Autodesk Inventor part; units mm, degrees
ref_plane "РабПлоскость4" through (-23, -29.9, -1) normal (0, -1, 0) x (1, 0, 0)
ref_plane "РабПлоскость8" through (0, 0, -1) normal (0, 0, -1) x (-1, 0, 0)
ref_plane "YZ Plane" through (0, 0, 0) normal (1, 0, 0) x (0, 1, 0)
sketch "Эскиз1" plane through (0, 0, 0) normal (0, 0, 1) x (1, 0, 0)
  line L0 (16.9838, 20.6364) -> (20.6364, 16.9838)
  arc A0 (16.9838, 20.6364) -> (16.3474, 20.9) centre (16.3474, 20) ccw
  line L1 (-16.3474, 20.9) -> (16.3474, 20.9)
  arc A1 (-16.3474, 20.9) -> (-16.9838, 20.6364) centre (-16.3474, 20) ccw
  line L2 (-20.6364, 16.9838) -> (-16.9838, 20.6364)
  arc A2 (-20.6364, 16.9838) -> (-20.9, 16.3474) centre (-20, 16.3474) ccw
  line L3 (-20.9, -16.3474) -> (-20.9, 16.3474)
  arc A3 (-20.9, -16.3474) -> (-20.6364, -16.9838) centre (-20, -16.3474) ccw
  line L4 (-16.9838, -20.6364) -> (-20.6364, -16.9838)
  arc A4 (-16.9838, -20.6364) -> (-16.3474, -20.9) centre (-16.3474, -20) ccw
  line L5 (16.3474, -20.9) -> (-16.3474, -20.9)
  arc A5 (16.3474, -20.9) -> (16.9838, -20.6364) centre (16.3474, -20) ccw
  line L6 (20.6364, -16.9838) -> (16.9838, -20.6364)
  arc A6 (20.6364, -16.9838) -> (20.9, -16.3474) centre (20, -16.3474) ccw
  line L7 (20.9, 16.3474) -> (20.9, -16.3474)
  arc A7 (20.9, 16.3474) -> (20.6364, 16.9838) centre (20, 16.3474) ccw
  circle A8 centre (15.5574, -15.5574) radius 1.45
  circle A9 centre (0, 0) radius 11
  circle A10 centre (-15.5574, -15.5574) radius 1.45
  circle A11 centre (-15.5574, 15.5574) radius 1.45
  circle A12 centre (15.5574, 15.5574) radius 1.45
  point P0 (0, 0)
extrude "Выдавливание1" add sketch "Эскиз1" along normal blind 3
sketch "Эскиз2" plane through (0, 0, 3) normal (0, 0, 1) x (1, 0, 0)
  line L0 (16.3474, 20.9) -> (-16.3474, 20.9) construction
  line L1 (-30, -20.9) -> (30, -20.9)
  line L2 (30, -20.9) -> (30, 20.9)
  line L3 (30, 20.9) -> (-30, 20.9)
  line L4 (-30, 20.9) -> (-30, -20.9)
  circle A0 centre (0, 0) radius 11 construction
  line L5 (-30, -20.9) -> (30, 20.9) construction
  line L6 (30, -20.9) -> (-30, 20.9) construction
  line L7 (-30, -20.9) -> (30, -20.9)
  line L8 (30, -20.9) -> (30, -48.9)
  line L9 (30, -48.9) -> (-30, -48.9)
  line L10 (-30, -48.9) -> (-30, -20.9)
  line L11 (-16.9838, 20.6364) -> (-20.6364, 16.9838)
  arc A1 (-20.6364, 16.9838) -> (-20.9, 16.3474) centre (-20, 16.3474) ccw
  line L12 (-20.9, 16.3474) -> (-20.9, -16.3474)
  arc A2 (-20.9, -16.3474) -> (-20.6364, -16.9838) centre (-20, -16.3474) ccw
  line L13 (-20.6364, -16.9838) -> (-16.9838, -20.6364)
  arc A3 (-16.9838, -20.6364) -> (-16.3474, -20.9) centre (-16.3474, -20) ccw
  line L14 (-16.3474, -20.9) -> (16.3474, -20.9)
  arc A4 (16.3474, -20.9) -> (16.9838, -20.6364) centre (16.3474, -20) ccw
  line L15 (16.9838, -20.6364) -> (20.6364, -16.9838)
  arc A5 (20.6364, -16.9838) -> (20.9, -16.3474) centre (20, -16.3474) ccw
  line L16 (20.9, -16.3474) -> (20.9, 16.3474)
  arc A6 (20.9, 16.3474) -> (20.6364, 16.9838) centre (20, 16.3474) ccw
  line L17 (20.6364, 16.9838) -> (16.9838, 20.6364)
  arc A7 (16.9838, 20.6364) -> (16.3474, 20.9) centre (16.3474, 20) ccw
  line L18 (16.3474, 20.9) -> (-16.3474, 20.9)
  arc A8 (-16.3474, 20.9) -> (-16.9838, 20.6364) centre (-16.3474, 20) ccw
  circle A9 centre (0, 0) radius 11 construction
  circle A10 centre (15.5574, 15.5574) radius 1.45 construction
  circle A11 centre (-15.5574, 15.5574) radius 1.45 construction
  circle A12 centre (-15.5574, -15.5574) radius 1.45 construction
  circle A13 centre (15.5574, -15.5574) radius 1.45 construction
  dimension "d4" = 60
  dimension "d5" = 60
  dimension "d6" = 28
extrude "Выдавливание2" add sketch "Эскиз2" against normal blind 8
ref_plane "РабПлоскость4" through (-23, -29.9, -1) normal (0, -1, 0) x (1, 0, 0)
chamfer "Фаска1" distance 4 angle 45 2 edges at (30, -48.9, -1) (-30, -48.9, -1)
chamfer "Фаска2" distance 8 angle 45 2 edges at (30, 20.9, -1) (-30, 20.9, -1)
sketch "Эскиз14" plane through (-30, -44.9, -5) normal (-1, 0, 0) x (0, 0, 1)
  line L0 (0, 57.8) -> (8, 57.8) construction
  line L1 (0, 0) -> (0, 57.8) construction
  line L2 (8, 0) -> (0, 0) construction
  line L3 (8, 57.8) -> (8, 0) construction
  line L4 (8, 57.8) -> (0, 57.8)
  line L5 (4, 57.8) -> (4, 0) construction
  line L6 (8, 0) -> (0, 0)
  circle A0 centre (4, 47.8) radius 2
  circle A1 centre (4, 33.8) radius 2
  dimension "d107" = 4
  dimension "d108" = 4
  dimension "d109" = 10
  dimension "d113" = 14
extrude "Выдавливание13" cut sketch "Эскиз14" against normal blind 6
sketch "Эскиз25" plane through (0, 0, 3) normal (0, 0, 1) x (1, 0, 0)
  line L0 (-20, -42.7) -> (20, -42.7)
  line L1 (20, -42.7) -> (20, -45.9)
  line L2 (20, -45.9) -> (-20, -45.9)
  line L3 (-20, -45.9) -> (-20, -42.7)
  line L4 (-20, -42.7) -> (20, -45.9) construction
  line L5 (20, -42.7) -> (-20, -45.9) construction
  line L6 (-26, -48.9) -> (26, -48.9) construction
  line L7 (26, -48.9) -> (-26, -48.9)
  line L8 (0, -48.9) -> (0, 20.9) construction
  line L9 (16.3474, 20.9) -> (-16.3474, 20.9) construction
  point P0 (0, 0)
  point P1 (0, -44.3)
  dimension "d170" = 40
  dimension "d171" = 3.2
  dimension "d172" = 3
extrude "Выдавливание25" cut sketch "Эскиз25" against normal blind 8
sketch "Эскиз27" plane through (-26, -48.9, 3) normal (0, -1, 0) x (1, 0, 0)
  line L0 (0, -8) -> (0, 0) construction
  line L1 (52, 0) -> (52, -8) construction
  line L2 (0, -4) -> (52, -4) construction
  circle A0 centre (16, -4) radius 1.1
  line L3 (46, 0) -> (46, -8) construction
  line L4 (6, 0) -> (46, 0) construction
  line L5 (46, 0) -> (46, -8) construction
  line L6 (46, -8) -> (6, -8) construction
  line L7 (6, -8) -> (6, 0) construction
  line L8 (6, 0) -> (46, -8) construction
  line L9 (46, 0) -> (6, -8) construction
  circle A1 centre (36, -4) radius 1.1
  point P0 (26, -4)
  dimension "d177" = 2.2
  dimension "d178" = 10
  dimension "d179" = 2.2
  dimension "d180" = 10
extrude "Выдавливание26" cut sketch "Эскиз27" against normal blind 14
sketch "Эскиз28" plane through (0, 0, 3) normal (0, 0, 1) x (1, 0, 0)
  line L0 (20, -45.9) -> (-20, -45.9) construction
  line L1 (-20, -45.9) -> (-20, -42.7) construction
  line L2 (-20, -42.7) -> (20, -42.7) construction
  line L3 (20, -42.7) -> (20, -45.9) construction
  line L4 (-26, -48.9) -> (26, -48.9)
  line L5 (-13, -48.9) -> (-7, -48.9)
  line L6 (-7, -48.9) -> (-7, -38.9)
  line L7 (-7, -38.9) -> (-13, -38.9)
  line L8 (-13, -38.9) -> (-13, -48.9)
  line L9 (-10, -38.9) -> (-10, -48.9) construction
  point P0 (0, 0)
  point P1 (-10, -43.9)
  point P2 (-20, -44.3)
  dimension "d183" = 6
  dimension "d184" = 10
  dimension "d185" = 10
extrude "Выдавливание27" cut sketch "Эскиз28" against normal blind 1.5
ref_plane "РабПлоскость8" through (0, 0, -1) normal (0, 0, -1) x (-1, 0, 0)
mirror "Зеркальное отражение4" about plane through (0, 0, 0) normal (1, 0, 0) of "Выдавливание27"
mirror "Зеркальное отражение5" about plane through (0, 0, -1) normal (0, 0, -1) of "Выдавливание27", "Зеркальное отражение4"
sketch "Эскиз29" plane through (0, 0, 1.5) normal (0, 0, 1) x (1, 0, 0)
  line L0 (-13, -38.9) -> (-7, -38.9) construction
  line L1 (-13, -42.7) -> (-13, -38.9) construction
  line L2 (7, -42.7) -> (7, -38.9) construction
  line L3 (7, -38.9) -> (13, -38.9) construction
  line L4 (-13, -38.9) -> (-7, -38.9)
  line L5 (-10, -38.9) -> (-10, -42.7) construction
  line L6 (-12, -39.9) -> (-8, -39.9)
  line L7 (-8, -39.9) -> (-8, -41.5)
  line L8 (-8, -41.5) -> (-12, -41.5)
  line L9 (-12, -41.5) -> (-12, -39.9)
  line L10 (-12, -39.9) -> (-8, -41.5) construction
  line L11 (-8, -39.9) -> (-12, -41.5) construction
  line L12 (-13, -42.7) -> (-7, -42.7)
  line L13 (7, -48.9) -> (-7, -48.9) construction
  line L14 (0, -48.9) -> (0, -38.1038) construction
  line L15 (12, -39.9) -> (8, -39.9)
  line L16 (8, -39.9) -> (8, -41.5)
  line L17 (8, -41.5) -> (12, -41.5)
  line L18 (12, -41.5) -> (12, -39.9)
  point P0 (0, 0)
  point P1 (-10, -40.7)
  dimension "d188" = 4
  dimension "d189" = 1.6
  dimension "d190" = 1.2
extrude "Выдавливание28" cut sketch "Эскиз29" against normal blind 10
properties part number "каретка_м2_без_м"
Check sheet for the modelled part. Datum: model origin and axes. Units: mm. A direction names the side the tool comes from. Give positions to 0.01 mm unless a question says otherwise; leave off trailing zeros. Loops run counter-clockwise (first coordinate to the right, second up) from the corner with the lowest first, then second, coordinate; pieces in that order, holes last. Notation, with made-up numbers: M 34,-5.75 L 40,-5.75 A28 cw 40,17.25 Z; hole C 47.5,87 d8. An arc over 180 degrees is marked long. Return JSON: item names as keys, results as strings. Group by question number.
1. Cross-section at A-A on x = -14. Record the boundary of the cut face in (y, z).
2. Tool access check on faces 4 (the flat face through (-7, -47, -4)), 5 (the flat face through (-8.7, -39.9, -1)), 6 (the flat face through (-10, -42, 1.5)). Record the directions out of +Z, -Z, +X, -X, +Y, -Y that give a thin tool (end or side, any length) a straight path to the whole face; none if there is none.
3. Mould release check, pull along Z, two halves, no side actions. Record for faces 1 (the flat face through (-10, -47, -3.5)), 2 (the flat face through (13, -47, -4)), 3 (the cylindrical face through (-8.95, -37.44, -0.67)): released by +Z, released by -Z, zero draft, split by the parting line, or undercut.
4. Cross-section at D-D on y = -12. Record the boundary of the cut face in (x, z), plus the area to 3 significant figures.
5. Thickness scan on L1, parallel to Z at x = 10, y = -37.4; L2, parallel to Z at x = 10, y = -48; L3, parallel to Y at x = 16, z = 0.5. Record the ranges inside material, lowest first.
6. Go/stop test with flat-tipped pins: pin 1 (1.6 mm diameter, centred on y = -47.5, z = -4, fed in from -X); pin 2 (1.1 mm diameter, centred on x = -9, y = -40, fed in from +Z); pin 3 (1.6 mm diameter, centred on y = -46.5, z = 2.5, fed in from -X). Record where each tip stops, or that it passes through.
7. Cross-section at C-C on x = 10. Record the boundary of the cut face in (y, z), plus the area to 3 significant figures.
8. Cross-section at B-B on y = 2.9. Record the boundary of the cut face in (x, z).
Return value:
{
 "1": {"outline": "M -48.9,-5 L -45.9,-5 L -45.9,3 L -48.9,3 Z; M -42.7,-5 L 20.9,-5 L 20.9,3 L -42.7,3 Z"},
 "2": {"face 4": "-Z, -Y", "face 5": "+Z, -Z", "face 6": "+Z, -Y"},
 "3": {"face 1": "released by -Z", "face 2": "zero draft", "face 3": "undercut"},
 "4": {"outline": "M -30,-5 L 30,-5 L 30,3 L -30,3 L -30,0.79 L -24,0.79 L -24,-2.79 L -30,-2.79 Z", "area": "459 mm^2"},
 "5": {"L1": "-5 to -2.1, 0.1 to 3", "L2": "-3.5 to -2.1, 0.1 to 1.5", "L3": "-48.9 to -45.9, -42.7 to 20.9"},
 "6": {"pin 1": "x = -28.2", "pin 2": "z = 1.5", "pin 3": "x = -29.2"},
 "7": {"outline": "M -48.9,-3.5 L -45.9,-3.5 L -45.9,-2.1 L -48.9,-2.1 Z; M -48.9,0.1 L -45.9,0.1 L -45.9,1.5 L -48.9,1.5 Z; M -42.7,-3.5 L -41.5,-3.5 L -41.5,-2.1 L -42.7,-2.1 Z; M -42.7,0.1 L -41.5,0.1 L -41.5,1.5 L -42.7,1.5 Z; M -39.9,-3.5 L -38.9,-3.5 L -38.9,-5 L 20.9,-5 L 20.9,3 L -38.9,3 L -38.9,1.5 L -39.9,1.5 L -39.9,0.1 L -34.9,0.1 L -34.9,-2.1 L -39.9,-2.1 Z", "area": "484 mm^2"},
 "8": {"outline": "M -30,-5 L 30,-5 L 30,3 L -30,3 L -30,1 L -24,1 L -24,-3 L -30,-3 Z"}
}
